The model under review builds one solid part; all positions refer to its coordinate system, in mm. Give positions to 0.01 mm unless a question says otherwise; leave off trailing zeros. Order: outer loops, then holes, each group sorted by start corner. A loop starts at its lowest first (then second) coordinate and runs counter-clockwise, first axis right, second up. Notation, with made-up numbers: M -22.5,-35 L 19.5,-35 A3 cw 19.5,-31 Z; hole C -33.75,31 d3. An arc over 180 degrees is marked long. One line per question, with ' | ' between items. Start each with the question number.
1. Wall thickness on L1, parallel to X at y = -18, z = 0; L2, parallel to X at y = 9, z = 6; L3, parallel to Z at x = -4, y = 8: over which ranges is each line inside the solid? List them lowest first.
2. Insertion check: P1, Ø8, axis at x = -6, y = 14.5, coming from the +Z side; P2, Ø1.5, axis at y = 10, z = -6, coming from the +X side; P3, Ø6, axis at y = -18, z = 3.5, coming from the +X side; P4, Ø1.5, axis at y = 4, z = 0.5, coming from the -X side. Each pin has a flat end and moves straight along its axis. Give the tip position at first contact, or say it passes through.
3. We need section B-B on y = -24. Write out the cut boundary in (x, z).
4. We need section A-A on y = 16. Write out the cut boundary in (x, z).
```python
from build123d import *
from build123d.topology import SkipClean

# Parameters (mm, degrees)
SKETCH_608_R        = 8
EXTRUDE_1_DEPTH     = 22
EXTRUDE_2_OUTLINE_W = 8
EXTRUDE_2_OUTLINE_H = 1


# Read off the part's stored shape, not the designer's step: 凸台-拉伸2
with BuildPart() as part:
    # Sketch 608 → 凸台-拉伸1 (new body)
    with BuildSketch(Plane(origin=(0, 0, 0), x_dir=(1, 0, 0), z_dir=(0, 1, 0))):
        with Locations(Location((0, 0, 0), (0, 0, 270))):
            Circle(SKETCH_608_R)
    extrude(amount=EXTRUDE_1_DEPTH)

    # 凸台-拉伸2 outline → 凸台-拉伸2 (revolve)
    with SkipClean():  # the faces are left unmerged after this step: merging them gives an invalid solid
        with BuildSketch(Plane.XY):
            with Locations((4, 22.5)):
                Rectangle(EXTRUDE_2_OUTLINE_W, EXTRUDE_2_OUTLINE_H)
            Polygon((8, 0), (0, 0), (0, -18), (7.056659973, -18), align=None)
        revolve(axis=Axis((0, 0, 0), (0, 1, 0)))
    add(part.part.scale(1), mode=Mode.REPLACE)  # the faces are merged on a copy

    # 草图7 → 旋转4 (revolve)
    with BuildSketch(Plane.XY, mode=Mode.PRIVATE) as revolve_4_sk:
        with BuildLine():
            Line((0, -18), (7.056659973, -18))
            Line((7.056659973, -18), (5.315312922, -32.182133633))
            ThreePointArc((5.315312922, -32.182133633), (3.880886548, -34.908529724), (1, -36))
            Line((1, -36), (0, -36))
            Line((0, -36), (0, -18))
        make_face()
    revolve(revolve_4_sk.sketch.rotate(Axis((0, -18, 0), (0, -1, 0)), 90), axis=Axis((0, -18, 0), (0, -1, 0)))


solid = part.part
```
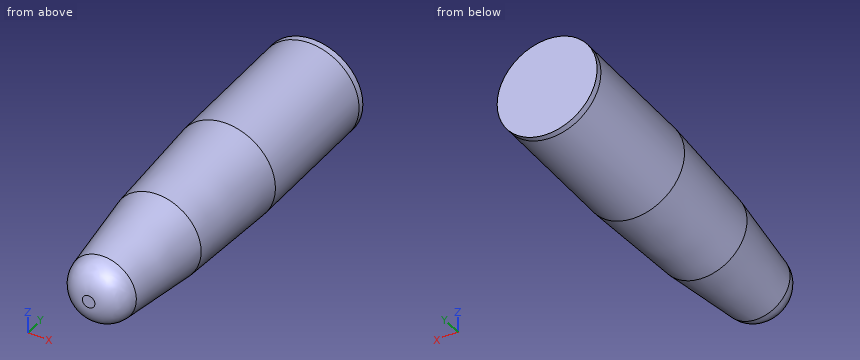
Entries:
1) L1: x = -7.06 to 7.06 | L2: x = -5.29 to 5.29 | L3: z = -6.93 to 6.93
2) P1: stops at z = 7.75 | P2: stops at x = 6.04 | P3: stops at x = 7.08 | P4: stops at x = -8
3) outline: C 0,0 d12.64
4) outline: C 0,0 d16
